The listing builds one solid part. Answer for the finished solid, in the listing's coordinates (mm). Face numbers are marked on the shaded views. Round coordinates to 2 decimals unless told otherwise and drop trailing zeros. Loops run counter-clockwise (first coordinate to the right, second up) from the corner with the lowest first, then second, coordinate; pieces in that order, holes last. Notation, with made-up numbers: M 72,-12 L 126,-12 A21 cw 126,19 Z; hole C 2.5,-14 d1. An arc over 180 degrees is marked long. Put each result on its own line as item: value. Start each with the question number.
(1) Determine the mould class of the marked faces 1, 2 and 3 for opening direction Y: released by +Y, released by -Y, zero draft, split by the parting line, or undercut.
(2) Section D-D, the plane x = 11.5 is taken. Determine the outline of the cut face in (y, z), then the cut area to 3 significant figures.
(3) Section A-A, the plane y = 32 is taken. Determine the outline of the cut face in (x, z), then the cut area to 3 significant figures.
(4) Flat-ended cylindrical pins translate along their axes: P1, Ø1.5, axis at y = 8, z = -8.5, coming from the -X side; P2, Ø6.5, axis at x = 1.5, y = 47, coming from the -Z side; P3, Ø5, axis at x = 9.5, z = -3, coming from the +Y side. Find the tip coordinate at first contact, or state that the pin passes through.
(5) Section B-B, the plane x = 3 is taken. Determine the outline of the cut face in (y, z).
(6) Straight lines are drawn through the part: line 1 (Y direction, x = -28.5, z = -8); line 2 (X direction, y = 6.5, z = -9); line 3 (Z direction, x = 6.5, y = 42). For each, find the intervals that lie inside material, in ascending order.
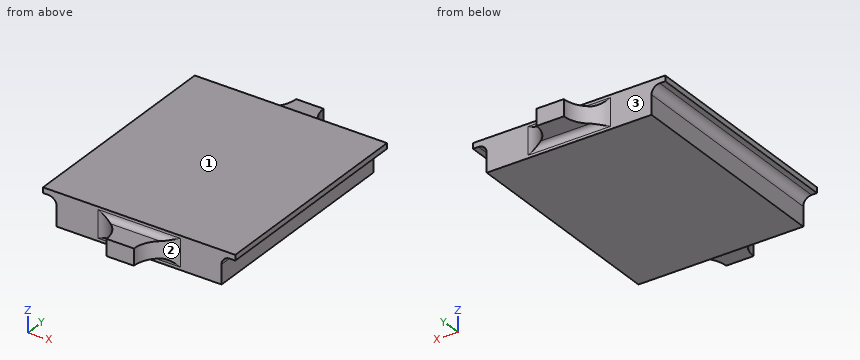
Autodesk Inventor part; units mm, degrees
ref_plane "YZ Plane" through (0, 0, 0) normal (1, 0, 0) x (0, 1, 0)
ref_plane "XZ Plane" through (0, 0, 0) normal (0, 1, 0) x (-1, 0, 0)
ref_plane "XY Plane" through (0, 0, 0) normal (0, 0, 1) x (1, 0, 0)
sketch "Esboço1" plane through (0, 0, 0) normal (0, 0, 1) x (1, 0, 0)
  line L0 (-30, -40) -> (30, -40)
  line L1 (30, -40) -> (30, 40)
  line L2 (30, 40) -> (-30, 40)
  line L3 (-30, 40) -> (-30, -40)
  line L4 (-30, -40) -> (30, 40) construction
  line L5 (30, -40) -> (-30, 40) construction
  line L6 (35, 40) -> (35, -40)
  line L7 (-35, -40) -> (-35, 40)
  line L8 (30, -40) -> (35, -40)
  line L9 (-35, -40) -> (-30, -40)
  line L10 (-35, 40) -> (-30, 40)
  line L11 (30, 40) -> (35, 40)
  point P0 (0, 0)
  dimension "d0" = 60
  dimension "d1" = 80
  dimension "d2" = 5
  dimension "d3" = 5
extrude "Extrusão1" add sketch "Esboço1" along normal blind 2
extrude "Extrusão2" add sketch "Esboço1" against normal blind 10 contours L3 L2 L1 L0
fillet "Arredondamento1" radius 3 2 edges at (30, 0, 0) (-30, 0, 0)
sketch "Esboço2" plane through (-35, -40, 2) normal (0, -1, 0) x (1, 0, 0)
  line L0 (65, -12) -> (5, -12)
  line L1 (65, -12) -> (65, 0)
  line L2 (0, 0) -> (70, 0)
  line L3 (65, -6) -> (5, -6) construction
  line L4 (5, -5) -> (5, -12)
  line L5 (40, -3) -> (30, -3)
  line L6 (30, -3) -> (30, -9)
  line L7 (30, -9) -> (40, -9)
  line L8 (40, -9) -> (40, -3)
  line L9 (40, -3) -> (30, -9) construction
  line L10 (30, -3) -> (40, -9) construction
  point P0 (35, -2)
  point P1 (35, -6)
  dimension "d9" = 10
  dimension "d10" = 6
extrude "Extrusão3" add sketch "Esboço2" along normal blind 10
fillet "Arredondamento2" radius 10 2 edges at (5, -40, -4) (-5, -40, -4)
fillet "Arredondamento3" radius 2 2 edges at (0, -40, -7) (0, -40, -1)
mirror "Espelhar1" about plane through (0, 0, 0) normal (0, 1, 0) of "Arredondamento2", "Extrusão3", "Arredondamento3"
properties part number "Repetidor"
Recorded:
1. face 1: zero draft
1. face 2: released by -Y
1. face 3: released by +Y
2. outline: M -40.63,-7.54 A2 cw -40,-9 L -40,-10 L 40,-10 L 40,-9 A2 cw 40.63,-7.54 L 40.63,-0.46 A2 cw 40,1 L 40,2 L -40,2 L -40,1 A2 cw -40.63,-0.46 Z
2. area: 970 mm²
3. outline: M -35,0 L -33,0 A3 cw -30,-3 L -30,-10 L 30,-10 L 30,-3 A3 cw 33,0 L 35,0 L 35,2 L -35,2 Z
3. area: 744 mm²
4. P1: stops at x = -30
4. P2: stops at z = -7
4. P3: stops at y = 44
5. outline: M -50,-7 L -42,-7 A2 cw -40,-9 L -40,-10 L 40,-10 L 40,-9 A2 cw 42,-7 L 50,-7 L 50,-1 L 42,-1 A2 cw 40,1 L 40,2 L -40,2 L -40,1 A2 cw -42,-1 L -50,-1 Z
6. line 1: y = -40 to 40
6. line 2: x = -30 to 30
6. line 3: z = -7 to -1
